Verification items for the finished model (mm, model axes). A direction names the side the tool comes from. Round coordinates to 2 decimals unless told otherwise and drop trailing zeros. Write each loop counter-clockwise with the first axis right and the second up, starting at its lowest first coordinate (ties: lowest second). Pieces come first, ordered by that corner, then holes.
from build123d import *

# Parameters (mm, degrees)
SKETCH1_R           = 5.25
BOSS_EXTRUDE1_DEPTH = 1
DOME1_FACE_RADIUS   = 5.25
DOME1_HEIGHT        = 1
SKETCH2_W           = 5
SKETCH2_H           = 9.233092656
BOSS_EXTRUDE2_DEPTH = 13
BOSS_EXTRUDE3_START = 1
SKETCH3_R           = 5.25
BOSS_EXTRUDE3_DEPTH = 1
BOSS_EXTRUDE4_DEPTH = 5


with BuildPart() as part:
    # Sketch1 → Boss-Extrude1 (new body)
    with BuildSketch(Plane.XY):
        Circle(SKETCH1_R)
    extrude(amount=BOSS_EXTRUDE1_DEPTH)

    # Dome1: a dome of height H over a round flat face of radius A is a cap of a sphere of radius (A * A + H * H) / (2 * H)
    dome1_r = (DOME1_FACE_RADIUS * DOME1_FACE_RADIUS + DOME1_HEIGHT * DOME1_HEIGHT) / (2 * DOME1_HEIGHT)
    dome1_base = Plane((0, 0, 1), z_dir=(0, 0, 1))
    with Locations(dome1_base.offset(DOME1_HEIGHT - dome1_r)):
        dome1_ball = Sphere(dome1_r, mode=Mode.PRIVATE)
    add(split(dome1_ball, bisect_by=dome1_base, keep=Keep.TOP, mode=Mode.PRIVATE))

    # Sketch2 → Boss-Extrude2 (add)
    with BuildSketch(Plane(origin=(0, 0, 0), x_dir=(-1, 0, 0), z_dir=(0, 0, -1))):
        Rectangle(SKETCH2_W, SKETCH2_H)
    extrude(amount=BOSS_EXTRUDE2_DEPTH)

    # Sketch3 → Boss-Extrude3 (add)
    with BuildSketch(Plane(origin=(0, 0, -13), x_dir=(-1, 0, 0), z_dir=(0, 0, -1)).offset(BOSS_EXTRUDE3_START)):
        with Locations(Location((0, 0, 0), (0, 0, 61.563109851))):
            Circle(SKETCH3_R)
    extrude(amount=-BOSS_EXTRUDE3_DEPTH)

    # Sketch4 → Boss-Extrude4 (add)
    with BuildSketch(Plane.XY.offset(-13)):
        Polygon((-4.3, 1.4), (-2.5, 2.15), (-2.5, 0.35), (-4.3, 1.1), align=None)
        Polygon((-4.3, -1.1), (-4.3, -1.4), (-2.5, -2.15), (-2.5, -0.35), align=None)
        Polygon((4.3, 1.4), (2.5, 2.15), (2.5, 0.35), (4.3, 1.1), align=None)
        Polygon((4.3, -1.1), (2.5, -0.35), (2.5, -2.15), (4.3, -1.4), align=None)
    extrude(amount=BOSS_EXTRUDE4_DEPTH)


solid = part.part
Q1. Material ranges on line 1 along Y through (x, z) = (0.25, -3.5); line 2 along X through (y, z) = (-3, -0.25); line 3 along Z through (x, y) = (-4.25, -1.5), recorded low to high.
Recorded:
line 1: y = -4.62 to 4.62
line 2: x = -2.5 to 2.5
line 3: z = -14 to -13, 0 to 1.27
Q2. Sectioned sample at D-D (x = 0). Enter the section's corners in (y, z).
Recorded:
outline: (-5.25, -14) - (5.25, -14) - (5.25, -13) - (4.62, -13) - (4.62, 0) - (5.25, 0) - (5.25, 1) arc R14.28 ccw to (-5.25, 1) - (-5.25, 0) - (-4.62, 0) - (-4.62, -13) - (-5.25, -13) - close
Q3. Tool access check on faces 1 (the flat face through (3.41, -0.73, -10.54)), 2 (the flat face through (4, 0, 0)), 3 (the flat face through (-2.5, 0, -5)), 4 (the flat face through (-3, 1, -8)). Record the directions out of +Z, -Z, +X, -X, +Y, -Y that give a thin tool (end or side, any length) a straight path to the whole face; none if there is none.
Recorded:
face 1: +X
face 2: +X, +Y, -Y
face 3: -X
face 4: -X, +Y, -Y
Q4. Sectioned sample at B-B (x = 4). Enter the section's corners in (y, z) (3 decimals), plus the area to 3 significant figures.
Recorded:
outline: (-3.4, -14) - (3.4, -14) - (3.4, -13) - (1.525, -13) - (1.525, -8) - (0.975, -8) - (0.975, -13) - (-0.975, -13) - (-0.975, -8) - (-1.525, -8) - (-1.525, -13) - (-3.4, -13) - close; (-3.4, 0) - (3.4, 0) - (3.4, 1) arc R13.71 ccw to (-3.4, 1) - close
area: 21.0 mm2
Q5. Sectioned sample at C-C (z = -11.75). Enter the section's corners in (x, y).
Recorded:
outline: (-4.3, -1.4) - (-2.5, -2.15) - (-2.5, -4.62) - (2.5, -4.62) - (2.5, -2.15) - (4.3, -1.4) - (4.3, -1.1) - (2.5, -0.35) - (2.5, 0.35) - (4.3, 1.1) - (4.3, 1.4) - (2.5, 2.15) - (2.5, 4.62) - (-2.5, 4.62) - (-2.5, 2.15) - (-4.3, 1.4) - (-4.3, 1.1) - (-2.5, 0.35) - (-2.5, -0.35) - (-4.3, -1.1) - close
Q6. Sectioned sample at A-A (y = 0). Enter the section's corners in (x, z).
Recorded:
outline: (-5.25, -14) - (5.25, -14) - (5.25, -13) - (2.5, -13) - (2.5, 0) - (5.25, 0) - (5.25, 1) arc R14.28 ccw to (-5.25, 1) - (-5.25, 0) - (-2.5, 0) - (-2.5, -13) - (-5.25, -13) - close
Q7. Release check for a two-part mould opening along Z. For faces 5 (the flat face through (4, 0, -13)), 6 (the flat face through (0, 0, -14)) record: released by +Z, released by -Z, zero draft, split by the parting line, or undercut.
Recorded:
face 5: undercut
face 6: released by -Z
Q8. Depth check by flat-ended pin: P1, Ø0.9, axis at x = -3.5, y = 1, coming from the +Z side; P2, Ø1, axis at y = -4, z = -5.5, coming from the -X side; P3, Ø3, axis at x = 4, y = 0.5, coming from the +Z side. Enter the tip coordinate at first touch or a pass-through.
Recorded:
P1: stops at z = 1.64
P2: stops at x = -2.5
P3: stops at z = 1.77
